Read the model definition and answer for the solid it produces. Units are mm, in the model's axes. Coordinates: 2 decimals unless noted, no trailing zeros. Order: outer loops, then holes, each group sorted by start corner. A loop starts at its lowest first (then second) coordinate and runs counter-clockwise, first axis right, second up.
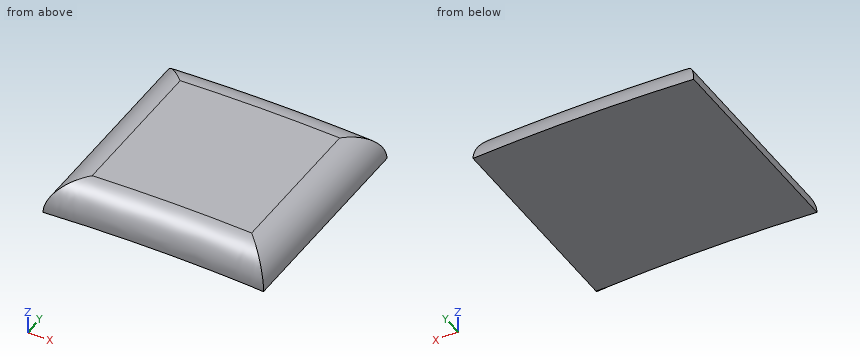
```python
from build123d import *

# Parameters (mm, degrees)
F0_R        = 316.25
F0_R_2      = 281.25
F1_DEPTH    = 10
F3_DEPTH    = 5
F4_W        = 212.0740879327
F4_H        = 34.9558026777
F4_W_2      = 196.2447150651
F4_H_2      = 35.0580604298
F5_DEPTH    = 84
F6_W        = 1.3297378083
F6_H        = 10.0317904726
F7_DEPTH    = 42
F8_T1_DEPTH = 60.0580604298
F8_T3_DEPTH = 60.0708356762
F8_T6_ANGLE = 12.4528096898
F8_T8_ANGLE = 11.0736814867


# Not quite as in the source:
# - a fillet or chamfer that OpenCascade refuses, or shapes differently, is made with other operations: its cross-section is extruded or revolved along the edge and cut away or added


with BuildPart() as f1:
    # F0 (on Top) → F1 (new body)
    with BuildSketch(Plane.XY):
        Circle(F0_R)
        Circle(F0_R_2, mode=Mode.SUBTRACT)
    extrude(amount=F1_DEPTH)

    # F2 (on face) → F3 (join)
    with BuildSketch(Plane.XY.offset(10)):
        with BuildLine():
            ThreePointArc((18.9455430955, 315.6820059757), (0.8957518585, 316.2487314261), (-17.1569601592, 315.7842637278))
            Line((-17.1569601592, 315.7842637278), (-17.1569601592, 280.726203298))
            ThreePointArc((-17.1569601592, 280.726203298), (0.8961391508, 281.2485723246), (18.9455430955, 280.6111702994))
            Line((18.9455430955, 280.6111702994), (18.9455430955, 315.6820059757))
        make_face()
    extrude(amount=F3_DEPTH)

    # F4 (on face) → F5 (cut)
    with BuildSketch(Plane.XY.offset(10)):
        Polygon((417.2187745571, -329.5601010323), (417.2187745571, 280.726203298), (231.0196310282, 280.726203298), (18.9455430955, 280.726203298), (-17.1569601592, 280.726203298), (-213.4016752243, 280.726203298), (-349.9614596367, 280.726203298), (-349.9614596367, -329.5601010323), align=None)
        with Locations((124.9825870618, 298.2041046368)):
            Rectangle(F4_W, F4_H)
        with Locations((-115.2793176918, 298.2552335129)):
            Rectangle(F4_W_2, F4_H_2)
    extrude(amount=-F5_DEPTH, mode=Mode.SUBTRACT)

    # F6 (on face) → F7 (cut)
    with BuildSketch(Plane.YZ.offset(18.9455430955)):
        Polygon((280.726203298, 10), (280.726203298, 0), (315.6820059757, 0), (315.6820059757, 10.0317904726), (280.726203298, 10.0317904726), align=None)
        with Locations((316.3468748798, 5.0158952363)):
            Rectangle(F6_W, F6_H)
    extrude(amount=-F7_DEPTH, mode=Mode.SUBTRACT)

    # F8: fillet of radius 5 on 4 edges, made by hand

    # F8_s2 → F8_t1 (cut)
    with BuildSketch(Plane.XZ.offset(-328.2842637278)):
        with BuildLine():
            ThreePointArc((-17.1569601592, 10), (-15.6924940651, 13.5355339059), (-12.1569601592, 15))
            Line((-12.1569601592, 15), (-17.1569601592, 15))
            Line((-17.1569601592, 15), (-17.1569601592, 10))
        make_face()
    extrude(amount=F8_T1_DEPTH, mode=Mode.SUBTRACT)

    # F8_s4 → F8_t3 (cut)
    with BuildSketch(Plane.XZ.offset(-328.1820059757)):
        with BuildLine():
            ThreePointArc((13.9455430955, 15), (17.4810770014, 13.5355339059), (18.9455430955, 10))
            Line((18.9455430955, 10), (18.9455430955, 15))
            Line((18.9455430955, 15), (13.9455430955, 15))
        make_face()
    extrude(amount=F8_T3_DEPTH, mode=Mode.SUBTRACT)

    # F8_s5 → F8_t6 (revolve, cut)
    with BuildSketch(Plane(origin=(0, 0, 0), x_dir=(0, 0, 1), z_dir=(-0.9944416157, -0.1052894726, 0))):
        with BuildLine():
            ThreePointArc((15, 286.25), (13.5355339059, 282.7144660941), (10, 281.25))
            Line((10, 281.25), (15, 281.25))
            Line((15, 281.25), (15, 286.25))
        make_face()
    revolve(axis=Axis((0, 0, 15), (0, 0, -1)), revolution_arc=F8_T6_ANGLE, mode=Mode.SUBTRACT)

    # F8_s7 → F8_t8 (revolve, cut)
    with BuildSketch(Plane(origin=(0, 0, 0), x_dir=(0, 0, 1), z_dir=(0.995057084, -0.0993045796, 0))):
        with BuildLine():
            ThreePointArc((10, -316.25), (13.5355339059, -314.7855339059), (15, -311.25))
            Line((15, -311.25), (15, -316.25))
            Line((15, -316.25), (10, -316.25))
        make_face()
    revolve(axis=Axis((0, 0, 15), (0, 0, 1)), revolution_arc=F8_T8_ANGLE, mode=Mode.SUBTRACT)


solid = f1.part
```
1) A cutting plane is placed at B-B, the plane z = 12. Determine the outline of the cut face in (x, y), and give its area (3 significant figures).
A:
outline: (-16.74, 281.17) arc R281.67 cw to (18.53, 281.06) - (18.53, 315.29) arc R315.83 ccw to (-16.74, 315.39) - close
area: 1,210 mm2
2) Straight lines are drawn through the part: line 1 (Z direction, x = 1, y = 292); line 2 (Z direction, x = -2, y = 313); line 3 (X direction, y = 301, z = 12.9). For each, find the intervals that lie inside material, in ascending order.
A:
line 1: z = 10.03 to 15
line 2: z = 10.03 to 14.68
line 3: x = -16.23 to 18.02
3) Flat-ended cylindrical pins translate along their axes: pin 1 Ø3 at (x, z) = (-5, 12.5) entering from +Y; pin 2 Ø3 at (x, y) = (-2.5, 299.5) entering from -Z; pin 3 Ø1.5 at (y, z) = (302, 14.5) entering from +X. Find the tip coordinate at first contact, or state that the pin passes through.
A:
pin 1: stops at y = 316.11
pin 2: stops at z = 10.03
pin 3: stops at x = 17.25
4) A cutting plane is placed at A-A, the plane y = 297.5. Determine the outline of the cut face in (x, z).
A:
outline: (-17.16, 10.03) - (18.95, 10.03) arc R5 ccw to (13.95, 15) - (-12.16, 15) arc R5 ccw to start
